```python
from build123d import *

# Parameters (mm, degrees)
EXTRUDE_1_DEPTH     = 2
SKETCH_7_R          = 1.1
CUT_EXTRUDE_5_DEPTH = 3.5
SKETCH_8_W          = 7.5
SKETCH_8_H          = 6
FILLET_1_RADIUS     = 3
FILLET_1_LENGTH     = 7.5
CUT_EXTRUDE_6_DEPTH = 10
SKETCH_12_R         = 1.1
CUT_EXTRUDE_7_DEPTH = 10


with BuildPart() as part:
    # 草图1 → 凸台-拉伸1 (new body)
    with BuildSketch(Plane(origin=(0, 0, 0), x_dir=(1, 0, 0), z_dir=(0, 1, 0))):
        with BuildLine():
            Line((-6.5, 3), (6.5, 3))
            ThreePointArc((6.5, 3), (9.5, 0), (6.5, -3))
            Line((6.5, -3), (-6.5, -3))
            ThreePointArc((-6.5, -3), (-9.5, 0), (-6.5, 3))
        make_face()
    extrude(amount=EXTRUDE_1_DEPTH)

    # 草图7 → 切除-拉伸5 (cut)
    with BuildSketch(Plane(origin=(0, 2, 0), x_dir=(1, 0, 0), z_dir=(0, 1, 0))):
        with Locations(Location((6.5, 0, 0), (0, 0, 270))):
            Circle(SKETCH_7_R)
        with Locations(Location((-6.5, 0, 0), (0, 0, 270))):
            Circle(SKETCH_7_R)
    extrude(amount=-CUT_EXTRUDE_5_DEPTH, mode=Mode.SUBTRACT)

    # 扫描1: sweep along a path in 草图9
    with BuildLine(Plane(origin=(0, 0, 0), x_dir=(0, 0, -1), z_dir=(1, 0, 0))) as sweep_1_path:
        Line((0, 2), (0, 4.566273071))
        ThreePointArc((0, 4.566273071), (-0.19369152, 5.94445985), (-0.759759519, 7.215869392))
        Line((-0.759759519, 7.215869392), (-5.299192642, 14.480480962))
    # 草图8 → 扫描1 (sweep)
    with BuildSketch(Plane(origin=(0, 2, 0), x_dir=(1, 0, 0), z_dir=(0, 1, 0))):
        Rectangle(SKETCH_8_W, SKETCH_8_H)
    sweep(path=sweep_1_path.line)

    # 圆角1: full round fillet: the end face becomes a half cylinder, R = half its width
    fillet_1_face = Plane((0, 14.480480962, 5.299192642), x_dir=(1, 0, 0), z_dir=(0, 0.848048096156, 0.529919264233))  # on the end face: x along it, z out of the body
    fillet_1_slab = fillet_1_face.offset(-FILLET_1_RADIUS / 2) * Box(FILLET_1_LENGTH, 2 * FILLET_1_RADIUS, FILLET_1_RADIUS, mode=Mode.PRIVATE)  # the body's end, R deep
    fillet_1_round = Plane((0, 11.936336674, 3.709434849), x_dir=(0, 0.848048096156, 0.529919264233), z_dir=(1, 0, 0)) * Cylinder(FILLET_1_RADIUS, FILLET_1_LENGTH, mode=Mode.PRIVATE)  # its axis R under the face
    add(fillet_1_slab - fillet_1_round, mode=Mode.SUBTRACT)

    # 草图10 → 切除-拉伸6 (cut)
    with BuildSketch(Plane(origin=(0, 0.095128767, -0.15223785), x_dir=(1, 0, 0), z_dir=(0, -0.5299192642332061, 0.8480480961564253))):
        with BuildLine():
            Line((1.372390297, 9.808736266), (2.069809275, 17.780271657))
            Line((2.069809275, 17.780271657), (-2.069809275, 17.780271657))
            Line((-2.069809275, 17.780271657), (-1.372390297, 9.808736266))
            ThreePointArc((-1.372390297, 9.808736266), (0, 7.538288577), (1.372390297, 9.808736266))
        make_face()
    extrude(amount=-CUT_EXTRUDE_6_DEPTH, mode=Mode.SUBTRACT)

    # 草图12 → 切除-拉伸7 (cut)
    with BuildSketch(Plane.ZY.offset(3.75)):
        with Locations((3.70943485, 11.936336673)):
            Circle(SKETCH_12_R)
    extrude(amount=-CUT_EXTRUDE_7_DEPTH, mode=Mode.SUBTRACT)


solid = part.part
```
Verification items for the finished model (mm, model axes). A direction names the side the tool comes from. Give positions to 0.01 mm unless a question says otherwise; leave off trailing zeros. Order: outer loops, then holes, each group sorted by start corner. A loop starts at its lowest first (then second) coordinate and runs counter-clockwise, first axis right, second up. Notation, with made-up numbers: (75, -12.75) -> (125, -12.75) arc R21 ccw to (125, 16.25) -> close; hole circle Ø8 at (52, 14). An arc over 180 degrees is marked (long way). One line per item, written item: value.
(1) Scan lines: line 1 along X through (y, z) = (0.6, 0); line 2 along Y through (x, z) = (-5, -2); line 3 along X through (y, z) = (9.5, 4.5). Record each from-to range of solid material in increasing order. Write a range as [from, to].
Final values:
line 1: [-9.5, -7.6], [-5.4, 5.4], [7.6, 9.5]
line 2: [0, 2]
line 3: [-3.75, -1.43], [1.43, 3.75]
(2) Tool access check on faces 4 (the face through (5, 2, 0)), 5 (the face through (0, 2, 3)), 6 (the face through (-5, 2, 0)). Record the directions out of +Z, -Z, +X, -X, +Y, -Y that give a thin tool (end or side, any length) a straight path to the whole face; none if there is none.
Final values:
face 4: +Z, -Z, +X, +Y
face 5: +Z, +X, -X, -Y
face 6: +Z, -Z, -X, +Y
(3) Sectioned sample at B-B on z = -2.25. Record the cut outline in (x, y).
Final values:
outline: (-8.48, 0) -> (8.48, 0) -> (8.48, 2) -> (3.75, 2) -> (3.75, 7.95) -> (-3.75, 7.95) -> (-3.75, 2) -> (-8.48, 2) -> close
(4) Sectioned sample at C-C on y = 11.25. Count the separate pieces of the cut face and the enclosed holes in it, then the cut area to 3 significant figures.
Final values:
separate pieces: 4
enclosed holes: 0
area: 23.2 mm^2
(5) Gauge pin test, flat ends, axial feed: pin 1 (5 mm diameter, centred on y = 5, z = 2, fed in from -X); pin 2 (2.5 mm diameter, centred on y = 11.94, z = 3.71, fed in from +X); pin 3 (3.5 mm diameter, centred on x = -6.5, z = 0, fed in from +Y); pin 4 (2 mm diameter, centred on x = 6.5, z = 0, fed in from -Y). Record the tip position at first contact, or that the pin passes through.
Final values:
pin 1: x = -3.75
pin 2: x = 3.75
pin 3: y = 2
pin 4: through
(6) Sectioned sample at A-A on z = 5.5. Record the cut outline in (x, y), then the cut area to 3 significant figures.
Final values:
outline: (-3.75, 9.14) -> (-1.45, 9.14) -> (-1.83, 14.34) -> (-3.75, 14.34) -> close; (1.45, 9.14) -> (3.75, 9.14) -> (3.75, 14.34) -> (1.83, 14.34) -> close
area: 22.0 mm^2
(7) Draft check along X on faces 1 (the face through (0.053, 5.11, 3.075)), 2 (the face through (9.5, 1, -0.1)), 3 (the face through (-1.607, 11.544, 5.086)). Enter one of: pulls with the +X half, pulls with the -X half, needs draft (parallel to the pull), parting line crosses it, or undercut.
Final values:
face 1: needs draft
face 2: pulls with the +X half
face 3: undercut
